The model under review builds one solid part; all positions refer to its coordinate system, in mm. Face numbers are marked on the shaded views. A direction names the side the tool comes from. Give positions to 0.01 mm unless a question says otherwise; leave off trailing zeros. Loops run counter-clockwise (first coordinate to the right, second up) from the corner with the lowest first, then second, coordinate; pieces in that order, holes last. Notation, with made-up numbers: (73.25, -38) - (131.25, -38) arc R31 ccw to (131.25, -10) - close; hole circle Ø6 at (26.5, -32). An arc over 180 degrees is marked (long way). Return JSON: item names as keys, results as strings. Group by question number.
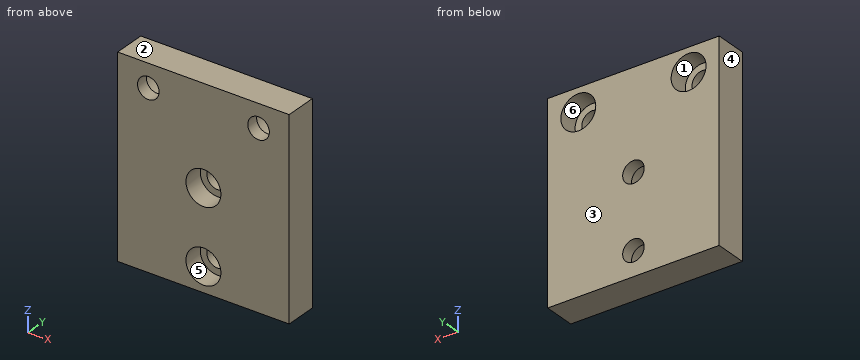
from build123d import *

# Parameters (mm, degrees)
F0_W           = 70
F0_H           = 80
F1_DEPTH       = 13
F4_D           = 8.8
F4_DEPTH       = 22.75
F4_CBORE_D     = 14.25
F4_CBORE_DEPTH = 8
F4_TIP         = 2.6437867237
F5_D           = 8.8
F5_DEPTH       = 22.75
F5_CBORE_D     = 14.25
F5_CBORE_DEPTH = 8
F5_TIP         = 2.6437867237


with BuildPart() as f1:
    # F0 (on Front) → F1 (new body)
    with BuildSketch(Plane.XZ):
        Rectangle(F0_W, F0_H)
    extrude(amount=F1_DEPTH)

    # F4
    with Locations(Plane(origin=(0, 0, 0), x_dir=(-1, 0, 0), z_dir=(0, 1, 0))):
        with Locations((-22.5, 30.5), (22.5, 30.5)):
            CounterBoreHole(F4_D / 2, F4_CBORE_D / 2, F4_CBORE_DEPTH, depth=F4_DEPTH)
            with Locations((0, 0, -(F4_DEPTH + F4_TIP / 2))):  # 118° drill point
                Cone(0, F4_D / 2, F4_TIP, mode=Mode.SUBTRACT)

    # F5
    with Locations(Plane.XZ.offset(13)):
        with Locations((0, 0), (0, -30)):
            CounterBoreHole(F5_D / 2, F5_CBORE_D / 2, F5_CBORE_DEPTH, depth=F5_DEPTH)
            with Locations((0, 0, -(F5_DEPTH + F5_TIP / 2))):  # 118° drill point
                Cone(0, F5_D / 2, F5_TIP, mode=Mode.SUBTRACT)


solid = f1.part
Item 1: For P1, Ø13, axis at x = 22.5, z = 30.5, coming from the +Y side; P2, Ø23, axis at x = -22.5, z = 30.5, coming from the -Y side; P3, Ø8, axis at x = 0, z = 0, coming from the +Y side; P4, Ø4.5, axis at x = 2.5, z = -2, coming from the -Y side, all flat-tipped, find the tip position at first contact; note any pin that passes through.
Item 2: Take a section at D-D (y = -10). State the section outline as (x, z) points (3 decimals).
Item 3: Tool access review of the marked faces 4, 5 and 6: name each direction out of +Z, -Z, +X, -X, +Y, -Y from which nothing blocks a thin tool from reaching the whole face with its end or side.
Item 4: Take a section at A-A (z = 30.5). State the section outline as (x, y) points (3 decimals).
Item 5: Take a section at C-C (x = -22.5). State the section outline as (y, z) points (3 decimals).
Item 6: Take a section at B-B (z = 0). State the section outline as (x, y) points (3 decimals).
Item 7: For L1, parallel to Z at x = 2, y = -7.75; L2, parallel to Z at x = 3.5, y = -3; L3, parallel to Z at x = -22.5, y = -4.25 (3 decimals), list the stretches that pass through material, from the lowest coordinate up. Write a range as from..to.
Item 8: Mouldability with a two-part tool opening along Z and no side actions: class the marked faces 1, 2 and 3 as +Z half, -Z half, draft (parallel to the pull), parting line (faces both ways), or undercut.
Check sheet entries:
{
 "1": {"P1": "stops at y = -8", "P2": "stops at y = -13", "P3": "passes through", "P4": "stops at y = -5"},
 "2": {"outline": "(-35, -40) - (35, -40) - (35, 40) - (-35, 40) - close; hole circle Ø8.8 at (-22.5, 30.5); hole circle Ø14.25 at (0, -30); hole circle Ø14.25 at (0, 0); hole circle Ø8.8 at (22.5, 30.5)"},
 "3": {"face 4": "+Z, -Z, -X, +Y, -Y", "face 5": "-Y", "face 6": "+Y"},
 "4": {"outline": "(-35, -13) - (-26.9, -13) - (-26.9, -8) - (-29.625, -8) - (-29.625, 0) - (-35, 0) - close; (-18.1, -13) - (18.1, -13) - (18.1, -8) - (15.375, -8) - (15.375, 0) - (-15.375, 0) - (-15.375, -8) - (-18.1, -8) - close; (26.9, -13) - (35, -13) - (35, 0) - (29.625, 0) - (29.625, -8) - (26.9, -8) - close"},
 "5": {"outline": "(-13, -40) - (0, -40) - (0, 23.375) - (-8, 23.375) - (-8, 26.1) - (-13, 26.1) - close; (-13, 34.9) - (-8, 34.9) - (-8, 37.625) - (0, 37.625) - (0, 40) - (-13, 40) - close"},
 "6": {"outline": "(-35, -13) - (-7.125, -13) - (-7.125, -5) - (-4.4, -5) - (-4.4, 0) - (-35, 0) - close; (4.4, -5) - (7.125, -5) - (7.125, -13) - (35, -13) - (35, 0) - (4.4, 0) - close"},
 "7": {"L1": "z = -40..-36.84, -23.16..-6.84, 6.84..40", "L2": "z = -40..-32.67, -27.33..-2.67, 2.67..40", "L3": "z = -40..23.375, 37.625..40"},
 "8": {"face 1": "undercut", "face 2": "+Z half", "face 3": "draft"}
}
